Input: part model. Units: mm. Frame: model coordinates. A direction names the side the tool comes from. Coordinates: 2 decimals unless noted, no trailing zeros. Write each loop counter-clockwise with the first axis right and the second up, starting at its lowest first coordinate (ties: lowest second). Pieces come first, ordered by that corner, then holes.
1) Pin query (flat end, axial travel): pin 1 Ø6 at (y, z) = (381.5, 0) entering from +X; pin 2 Ø3 at (x, z) = (104, 4.5) entering from +Y. Return the tip coordinate at first contact, or that it passes through.
2) Section query C-C (x = 102). Output: boundary loops of the cut face in (y, z), then the cut area to 3 significant figures.
3) Line query: L1, parallel to Y at x = 0, z = -0.75; L2, parallel to X at y = 102, z = 4.25; L3, parallel to X at y = 453, z = 0.25. Output: solid intervals per line, ascending.
4) Section query A-A (x = 0). Output: boundary loops of the cut face in (y, z), then the cut area to 3 significant figures.
5) Section query B-B (z = 2). Output: boundary loops of the cut face in (x, y), then the cut area to 3 significant figures.
6) Set-up query: faces 5 (the flat face through (50, 75, 3)), 6 (the flat face through (100.7, 283.488, 3.284)). Return all of +Z, -Z, +X, -X, +Y, -Y with unobstructed straight access to the full face (end or side cutting, diameter ignored); none if empty.
7) Draft query along Y for faces 1 (the cylindrical face through (-1.953, 440.128, 3.016)), 2 (the flat face through (50, 378, 3)), 3 (the cylindrical face through (-1.099, 504.988, 3.016)), 4 (the cylindrical face through (-14.985, -0.66, 3.016)). Return one class per face: pulls with the +Y half, pulls with the -Y half, needs draft (parallel to the pull), parting line crosses it, or undercut.
8) Section query D-D (y = 343.5). Output: boundary loops of the cut face in (x, z).
Autodesk Inventor part; units mm, degrees
ref_plane "YZ Plane" through (0, 0, 0) normal (1, 0, 0) x (0, 1, 0)
ref_plane "XZ Plane" through (0, 0, 0) normal (0, 1, 0) x (-1, 0, 0)
ref_plane "XY Plane" through (0, 0, 0) normal (0, 0, 1) x (1, 0, 0)
sketch "Sketch1" plane through (0, 0, 0) normal (0, 0, 1) x (1, 0, 0)
  line L0 (0, 0) -> (0, 455) construction
  line L1 (50, 0) -> (50, 455)
  line L2 (-50, 455) -> (-50, 0)
  arc A0 (-50, 0) -> (50, 0) centre (0, 0) ccw
  arc A1 (50, 455) -> (-50, 455) centre (0, 455) ccw
  circle A2 centre (0, 455) radius 15
  circle A3 centre (0, 0) radius 15
  point P0 (0, 227.5)
  point P1 (0, 505)
  point P2 (0, -50)
  dimension "d0" = 455
  dimension "d2" = 30
  dimension "d3" = 30
  dimension "d6" = 555
extrude "Extrusion1" add sketch "Sketch1" along normal blind 12.7 and the other way blind 6.4
sketch "Sketch3" plane through (0, 0, 12.7) normal (0, 0, 1) x (1, 0, 0)
  line L0 (50, 0) -> (50, 455)
  line L1 (150, 227.5) -> (150, 265)
  line L2 (150, 265) -> (50, 302.5)
  line L3 (150, 227.5) -> (150, 190)
  line L4 (150, 190) -> (50, 152.5)
  point P0 (0, 0)
  point P1 (50, 227.5)
  dimension "d9" = 150
  dimension "d10" = 75
  dimension "d11" = 152.5
  dimension "d12" = 100
extrude "Extrusion2" add sketch "Sketch3" against normal blind 19.1
sketch "Sketch4" plane through (0, 0, -6.4) normal (0, 0, -1) x (-1, 0, 0)
  point P0 (0, 0)
properties part number "Eslabon de arrastre externo" material "Steel, Mild"
Answer:
1. pin 1: stops at x = 50
1. pin 2: stops at y = 282.81
2. outline: (172, -6.4) - (283, -6.4) - (283, 12.7) - (172, 12.7) - close
2. area: 2,120 mm2
3. L1: y = -50 to -15, 15 to 440, 470 to 505
3. L2: x = -50 to 50
3. L3: x = -50 to -14.87, 14.87 to 50
4. outline: (-50, -6.4) - (-15, -6.4) - (-15, 12.7) - (-50, 12.7) - close; (15, -6.4) - (440, -6.4) - (440, 12.7) - (15, 12.7) - close; (470, -6.4) - (505, -6.4) - (505, 12.7) - (470, 12.7) - close
4. area: 9,450 mm2
5. outline: (-50, 0) arc R50 ccw to (50, 0) - (50, 152.5) - (150, 190) - (150, 265) - (50, 302.5) - (50, 455) arc R50 ccw to (-50, 455) - close; hole circle Ø30 at (0, 0); hole circle Ø30 at (0, 455)
5. area: 63,200 mm2
6. face 5: +Z, -Z, +X, -Y
6. face 6: +Z, -Z, +X, +Y
7. face 1: undercut
7. face 2: needs draft
7. face 3: pulls with the +Y half
7. face 4: undercut
8. outline: (-50, -6.4) - (50, -6.4) - (50, 12.7) - (-50, 12.7) - close
